```python
from build123d import *

# Parameters (mm, degrees)
SKETCH_1_R          = 2.05
EXTRUDE_1_DEPTH     = 3
SKETCH_2_R          = 1.5
CUT_EXTRUDE_1_DEPTH = 3


with BuildPart() as part:
    # Эскиз1 → Бобышка-Вытянуть1 (new body)
    with BuildSketch(Plane(origin=(0, 0, 0), x_dir=(1, 0, 0), z_dir=(0, 1, 0))):
        with BuildLine():
            Line((-14, -22.5), (14, -22.5))
            ThreePointArc((14, -22.5), (20.01040764, -20.01040764), (22.5, -14))
            Line((22.5, -14), (22.5, 14))
            ThreePointArc((22.5, 14), (20.01040764, 20.01040764), (14, 22.5))
            Line((14, 22.5), (-14, 22.5))
            ThreePointArc((-14, 22.5), (-20.01040764, 20.01040764), (-22.5, 14))
            Line((-22.5, 14), (-22.5, -14))
            ThreePointArc((-22.5, -14), (-20.01040764, -20.01040764), (-14, -22.5))
        make_face()
        with Locations(Location((14, 14, 0), (0, 0, 270))):
            Circle(SKETCH_1_R, mode=Mode.SUBTRACT)
        with Locations(Location((14, -14, 0), (0, 0, 270))):
            Circle(SKETCH_1_R, mode=Mode.SUBTRACT)
        with Locations(Location((-14, -14, 0), (0, 0, 270))):
            Circle(SKETCH_1_R, mode=Mode.SUBTRACT)
        with Locations(Location((-14, 14, 0), (0, 0, 270))):
            Circle(SKETCH_1_R, mode=Mode.SUBTRACT)
    extrude(amount=EXTRUDE_1_DEPTH)

    # Эскиз2 → Вырез-Вытянуть1 (cut)
    with BuildSketch(Plane.XZ):
        with Locations(Location((0, 2.5, 0), (0, 0, 270))):
            Circle(SKETCH_2_R)
    extrude(amount=-CUT_EXTRUDE_1_DEPTH, mode=Mode.SUBTRACT)


solid = part.part
```
For this review, take the finished solid that the model builds, in its own axes (mm). Round coordinates to 2 decimals unless told otherwise and drop trailing zeros. Write each loop counter-clockwise with the first axis right and the second up, starting at its lowest first coordinate (ties: lowest second). Pieces come first, ordered by that corner, then holes. Notation, with made-up numbers: (-12.5, 73) - (9.5, 73) arc R8 ccw to (9.5, 79) - close; hole circle Ø10 at (-32, -1). An arc over 180 degrees is marked (long way). Answer as CSV lines item,"result". Start each with the question number.
(1) Add section A-A, the plane y = 1.3. State the section outline as (x, z) points, plus the area to 3 significant figures.
(2) For pin 1 (3.5 mm diameter, centred on x = 14, z = 14, fed in from +Y); pin 2 (1 mm diameter, centred on y = 0.5, z = 15.5, fed in from -X), all flat-tipped, find the tip position at first contact; note any pin that passes through.
(3) Add section B-B, the plane x = -19. State the section outline as (y, z) points.
(4) Add section C-C, the plane z = 18. State the section outline as (x, y) points, plus the area to 3 significant figures.
(5) For line 1 (X direction, y = 1.4, z = 14); line 2 (X direction, y = 2, z = 2.5); line 3 (Z direction, x = 13, y = 1.45), list the stretches that pass through material, from the lowest coordinate up.
(6) Mouldability with a two-part tool opening along Z and no side actions: class faces 1 (the flat face through (0, 1, 22.5)), 2 (the flat face through (22.5, 1, 0)), 3 (the cylindrical face through (-16.001, 1.479, -14.444)) as +Z half, -Z half, draft (parallel to the pull), parting line (faces both ways), or undercut.
From the geometry:
1,outline,"(-22.5, -14) arc R8.5 ccw to (-14, -22.5) - (14, -22.5) arc R8.5 ccw to (22.5, -14) - (22.5, 14) arc R8.5 ccw to (14, 22.5) - (-14, 22.5) arc R8.5 ccw to (-22.5, 14) - close; hole circle Ø4.1 at (-14, -14); hole circle Ø4.1 at (-14, 14); hole circle Ø3 at (0, 2.5); hole circle Ø4.1 at (14, -14); hole circle Ø4.1 at (14, 14)"
1,area,"1,900 mm²"
2,pin 1,"passes through"
2,pin 2,"stops at x = -22.44"
3,outline,"(0, -20.87) - (3, -20.87) - (3, 20.87) - (0, 20.87) - close"
4,outline,"(-21.5, 0) - (21.5, 0) - (21.5, 3) - (-21.5, 3) - close"
4,area,"129 mm²"
5,line 1,"x = -22.5 to -16.05, -11.95 to 11.95, 16.05 to 22.5"
5,line 2,"x = -22.5 to -1.5, 1.5 to 22.5"
5,line 3,"z = -22.5 to -15.79, -12.21 to 12.21, 15.79 to 22.5"
6,face 1,"+Z half"
6,face 2,"draft"
6,face 3,"undercut"
